Geometry: final body of the model. Coordinates: model frame, mm. A direction names the side the tool comes from. Coordinates: 2 decimals unless noted, no trailing zeros. Write each loop counter-clockwise with the first axis right and the second up, starting at its lowest first coordinate (ties: lowest second). Pieces come first, ordered by that corner, then holes. Notation, with made-up numbers: (65, 74) - (116, 74) arc R21 ccw to (116, 100) - close; hole circle Ø8 at (26.25, 42.25). An arc over 180 degrees is marked (long way). Put each result on its own line as item: value.
```python
from build123d import *

# Parameters (mm, degrees)
SKETCH1_W           = 16
SKETCH1_H           = 25
BOSS_EXTRUDE1_DEPTH = 12.5
CUT_EXTRUDE1_DEPTH  = 6.056
SKETCH4_W           = 5
SKETCH4_H           = 25
BOSS_EXTRUDE2_DEPTH = 6
SKETCH3_R           = 1.7145
CUT_EXTRUDE2_DEPTH  = 5
SKETCH6_R           = 0.5
CUT_EXTRUDE3_DEPTH  = 4
SKETCH7_R           = 1.5
CUT_EXTRUDE4_DEPTH  = 2


with BuildPart() as part:
    # Sketch1 → Boss-Extrude1 (new body)
    with BuildSketch(Plane(origin=(0, 0, 0), x_dir=(1, 0, 0), z_dir=(0, 1, 0))):
        with Locations((8, 12.5)):
            Rectangle(SKETCH1_W, SKETCH1_H)
    extrude(amount=BOSS_EXTRUDE1_DEPTH)

    # Sketch2 → Cut-Extrude1 (cut)
    with BuildSketch(Plane(origin=(0, 12.5, 0), x_dir=(1, 0, 0), z_dir=(0, 1, 0))):
        Polygon((4, 23.098280204), (6.4, 23.098280204), (6.4, 25), (8.6, 25), (8.6, 23.098280204), (11, 23.098280204), (11, 3.280280204), (8.6, 3.280280204), (8.6, 1.605280204), (6.4, 1.605280204), (6.4, 3.280280204), (4, 3.280280204), align=None)
    extrude(amount=-CUT_EXTRUDE1_DEPTH, mode=Mode.SUBTRACT)

    # Sketch4 → Boss-Extrude2 (add)
    with BuildSketch(Plane(origin=(0, 12.5, 0), x_dir=(1, 0, 0), z_dir=(0, 1, 0))):
        with Locations((13.5, 12.5)):
            Rectangle(SKETCH4_W, SKETCH4_H)
    extrude(amount=BOSS_EXTRUDE2_DEPTH)

    # Sketch3 → Cut-Extrude2 (cut)
    with BuildSketch(Plane(origin=(16, 0, 0), x_dir=(0, 0, -1), z_dir=(1, 0, 0))):
        with Locations((7.205280204, 14.644)):
            Circle(SKETCH3_R)
        with Locations((19.173280204, 14.644)):
            Circle(SKETCH3_R)
    extrude(amount=-CUT_EXTRUDE2_DEPTH, mode=Mode.SUBTRACT)

    # Sketch6 → Cut-Extrude3 (cut)
    with BuildSketch(Plane(origin=(0, 6.444, 0), x_dir=(1, 0, 0), z_dir=(0, 1, 0))):
        with Locations(Location((5.875, 9.605280204, 0), (0, 0, 270))):
            Circle(SKETCH6_R)
        with Locations(Location((9.125, 9.605280204, 0), (0, 0, 270))):
            Circle(SKETCH6_R)
        with Locations(Location((5.875, 17.605280204, 0), (0, 0, 270))):
            Circle(SKETCH6_R)
        with Locations(Location((9.125, 17.605280204, 0), (0, 0, 270))):
            Circle(SKETCH6_R)
    extrude(amount=-CUT_EXTRUDE3_DEPTH, mode=Mode.SUBTRACT)

    # Sketch7 → Cut-Extrude4 (cut)
    with BuildSketch(Plane(origin=(0, 6.444, 0), x_dir=(1, 0, 0), z_dir=(0, 1, 0))):
        with Locations(Location((7.5, 21.605280204, 0), (0, 0, 270))):
            Circle(SKETCH7_R)
        with Locations(Location((7.5, 13.605280204, 0), (0, 0, 270))):
            Circle(SKETCH7_R)
        with Locations(Location((7.5, 5.605280204, 0), (0, 0, 270))):
            Circle(SKETCH7_R)
    extrude(amount=-CUT_EXTRUDE4_DEPTH, mode=Mode.SUBTRACT)


solid = part.part
```
1. Section query D-D (z = -15.75). Return loops of the section in (x, y), then the cut area to 3 significant figures.
Answer below:
outline: (0, 0) - (16, 0) - (16, 18.5) - (11, 18.5) - (11, 6.44) - (4, 6.44) - (4, 12.5) - (0, 12.5) - close
area: 188 mm²
2. Mould query, pull axis Z, two halves, no side actions, for faces 4 (the flat face through (8, 4.444, -14)), 5 (the flat face through (10, 7, -25)), 6 (the flat face through (13, 18.5, -13)). Classes: +Z half, -Z half, draft (parallel to the pull), parting line (faces both ways), or undercut.
Answer below:
face 4: undercut
face 5: -Z half
face 6: draft
3. Section query B-B (y = 7). Return loops of the section in (x, z).
Answer below:
outline: (0, -25) - (6.4, -25) - (6.4, -23.1) - (4, -23.1) - (4, -3.28) - (6.4, -3.28) - (6.4, -1.61) - (8.6, -1.61) - (8.6, -3.28) - (11, -3.28) - (11, -23.1) - (8.6, -23.1) - (8.6, -25) - (16, -25) - (16, 0) - (0, 0) - close
4. Section query C-C (x = 7.5). Return loops of the section in (y, z), then the cut area to 3 significant figures.
Answer below:
outline: (0, -25) - (6.44, -25) - (6.44, -23.11) - (4.44, -23.11) - (4.44, -20.11) - (6.44, -20.11) - (6.44, -15.11) - (4.44, -15.11) - (4.44, -12.11) - (6.44, -12.11) - (6.44, -7.11) - (4.44, -7.11) - (4.44, -4.11) - (6.44, -4.11) - (6.44, -1.61) - (12.5, -1.61) - (12.5, 0) - (0, 0) - close
area: 153 mm²
5. Pin query (flat end, axial travel): pin 1 Ø1.5 at (x, z) = (7.5, -14.5) entering from +Y; pin 2 Ø0.7 at (x, y) = (8, 8) entering from -Z; pin 3 Ø2 at (y, z) = (14.64, -19.17) entering from +X; pin 4 Ø4 at (x, z) = (2, -20) entering from +Y. Return the tip coordinate at first contact, or that it passes through.
Answer below:
pin 1: stops at y = 6.44
pin 2: stops at z = -1.61
pin 3: passes through
pin 4: stops at y = 12.5
6. Ray query, probe 1 along Z at (x, y) = (12.25, 14.5); probe 2 along X at (y, z) = (6.75, -18.5); probe 3 along X at (y, z) = (6, -17.75). Return the intervals inside material, ascending. Write a range as from..to.
Answer below:
probe 1: z = -25..-20.88, -17.46..-8.91, -5.5..0
probe 2: x = 0..4, 11..16
probe 3: x = 0..5.4, 6.35..8.65, 9.6..16
7. Section query A-A (z = -8.5). Return loops of the section in (x, y).
Answer below:
outline: (0, 0) - (16, 0) - (16, 13.52) - (11, 13.52) - (11, 6.44) - (4, 6.44) - (4, 12.5) - (0, 12.5) - close; (11, 15.77) - (16, 15.77) - (16, 18.5) - (11, 18.5) - close
8. Set-up query: faces 1 (the flat face through (6.4, 10, -24)), 2 (the flat face through (10, 12.5, -24)), 3 (the flat face through (8, 4.444, -22)). Return all of +Z, -Z, +X, -X, +Y, -Y with unobstructed straight access to the full face (end or side cutting, diameter ignored); none if empty.
Answer below:
face 1: -Z, +Y
face 2: +Z, -Z, -X, +Y
face 3: +Y
